Read the model definition and answer for the solid it produces. Units are mm, in the model's axes. A direction names the side the tool comes from. Coordinates: 2 decimals unless noted, no trailing zeros. Write each loop counter-clockwise with the first axis right and the second up, starting at its lowest first coordinate (ties: lowest second). Pieces come first, ordered by that corner, then holes.
(1) The part is cut by section C-C, the plane y = 22.5. Determine the outline of the cut face in (x, z).
(2) Straight lines are drawn through the part: line 1 along Y through (x, z) = (-9.3, 0); line 2 along X through (y, z) = (20, -8); line 3 along Y through (x, z) = (-3, 13.5). For each, find the intervals that lie inside material, in ascending order.
(3) The part is cut by section B-B, the plane z = 0. Determine the outline of the cut face in (x, y).
(4) The part is cut by section A-A, the plane y = 11.5. Determine the outline of the cut face in (x, z), and give its area (3 significant figures).
(5) The part is cut by section D-D, the plane x = -5.5. Determine the outline of the cut face in (y, z).
(6) Determine the mould class of faces 1 (the flat face through (14, 2, 14)), 2 (the flat face through (8, 37.5, 0)), 3 (the flat face through (0, 7, 0)) for opening direction X: pulls with the +X half, pulls with the -X half, needs draft (parallel to the pull), parting line crosses it, or undercut.
(7) Given pin 1 (5 mm diameter, centred on x = -14, z = 7.5, fed in from +Y); pin 2 (4.5 mm diameter, centred on x = 0.5, z = 2, fed in from +Y); pin 3 (15 mm diameter, centred on y = 29, z = -4, fed in from -X), each flat-ended and moving along its own axis, determine where each tip first touches the part or whether it passes through.
(8) Which of the six approach directions +Z, -Z, +X, -X, +Y, -Y give full straight-line access (tool end or side, diameter ignored) to faces 4 (the flat face through (-4.5, 15, -3)), 5 (the flat face through (-13, 4.5, 0)), 6 (the flat face through (10.5, 13, 0))?
```python
from build123d import *

# Parameters (mm, degrees)
EXTRUDE_1_DEPTH     = 4.5
EXTRUDE_2_DEPTH     = 30
SKETCH_3_W          = 4.5
SKETCH_3_H          = 33
SKETCH_3_W_2        = 9
SKETCH_3_H_2        = 30.5
CUT_EXTRUDE_1_DEPTH = 30
SKETCH_4_R          = 7.5
CUT_EXTRUDE_2_DEPTH = 30


with BuildPart() as part:
    # 草图1 → 凸台-拉伸1 (new body)
    with BuildSketch(Plane(origin=(0, 0, 0), x_dir=(1, 0, 0), z_dir=(0, 1, 0))):
        Polygon((-15, 13), (-13, 15), (13, 15), (15, 13), (15, -13), (13, -15), (-13, -15), (-15, -13), align=None)
    extrude(amount=EXTRUDE_1_DEPTH)

    # 草图2 → 凸台-拉伸2 (add)
    with BuildSketch(Plane(origin=(15, 0, 0), x_dir=(0, 0, -1), z_dir=(1, 0, 0))):
        Polygon((-15, 4.5), (-15, 35.5), (-13, 37.5), (13, 37.5), (15, 35.5), (15, 4.5), align=None)
    extrude(amount=-EXTRUDE_2_DEPTH)

    # 草图3 → 切除-拉伸1 (cut)
    with BuildSketch(Plane.XY.offset(15)):
        with Locations((-12.75, 21)):
            Rectangle(SKETCH_3_W, SKETCH_3_H)
        with Locations((12.75, 21)):
            Rectangle(SKETCH_3_W, SKETCH_3_H)
        with Locations((0, 22.25)):
            Rectangle(SKETCH_3_W_2, SKETCH_3_H_2)
    extrude(amount=-CUT_EXTRUDE_1_DEPTH, mode=Mode.SUBTRACT)

    # 草图4 → 切除-拉伸2 (cut)
    with BuildSketch(Plane(origin=(10.5, 0, 0), x_dir=(0, 0, -1), z_dir=(1, 0, 0))):
        with Locations((0, 22.5)):
            Circle(SKETCH_4_R)
    extrude(amount=-CUT_EXTRUDE_2_DEPTH, mode=Mode.SUBTRACT)


solid = part.part
```
Computed:
1. outline: (-10.5, -15) - (-4.5, -15) - (-4.5, -7.5) - (-10.5, -7.5) - close; (-10.5, 7.5) - (-4.5, 7.5) - (-4.5, 15) - (-10.5, 15) - close; (4.5, -15) - (10.5, -15) - (10.5, -7.5) - (4.5, -7.5) - close; (4.5, 7.5) - (10.5, 7.5) - (10.5, 15) - (4.5, 15) - close
2. line 1: y = 0 to 15, 30 to 37.5
2. line 2: x = -10.5 to -4.5, 4.5 to 10.5
2. line 3: y = 0 to 7
3. outline: (-15, 0) - (15, 0) - (15, 4.5) - (10.5, 4.5) - (10.5, 15) - (4.5, 15) - (4.5, 7) - (-4.5, 7) - (-4.5, 15) - (-10.5, 15) - (-10.5, 4.5) - (-15, 4.5) - close; (-10.5, 30) - (-4.5, 30) - (-4.5, 37.5) - (-10.5, 37.5) - close; (4.5, 30) - (10.5, 30) - (10.5, 37.5) - (4.5, 37.5) - close
4. outline: (-10.5, -15) - (-4.5, -15) - (-4.5, 15) - (-10.5, 15) - close; (4.5, -15) - (10.5, -15) - (10.5, 15) - (4.5, 15) - close
4. area: 360 mm2
5. outline: (0, -15) - (35.5, -15) - (37.5, -13) - (37.5, 13) - (35.5, 15) - (0, 15) - close; hole circle Ø15 at (22.5, 0)
6. face 1: pulls with the +X half
6. face 2: needs draft
6. face 3: undercut
7. pin 1: stops at y = 4.5
7. pin 2: stops at y = 7
7. pin 3: stops at x = -10.5
8. face 4: +Z, -Z, +Y
8. face 5: +Z, -Z, -X, +Y
8. face 6: +Z, -Z, +X, +Y
